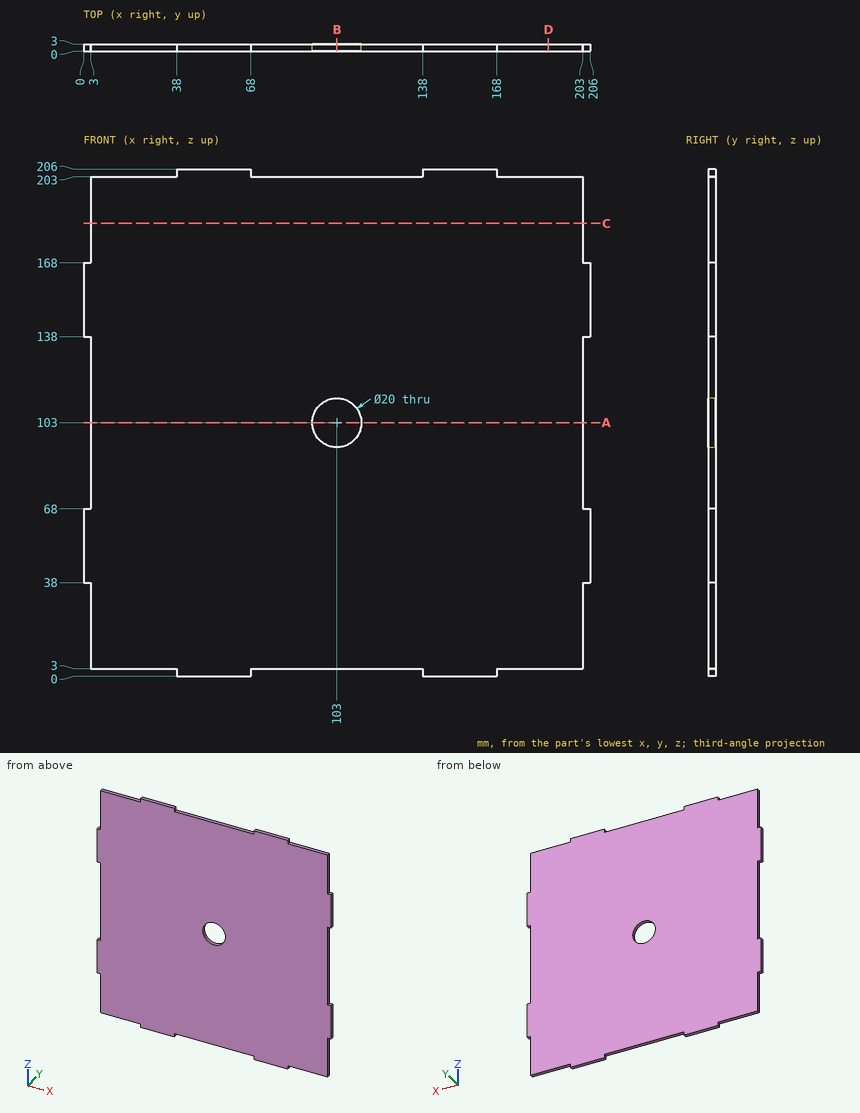
Job drawing, mm, ordinate dimensions from the low corner. One solid piece. Coordinates: 2 decimals unless noted, no trailing zeros. Order: outer loops, then holes, each group sorted by start corner. A loop starts at its lowest first (then second) coordinate and runs counter-clockwise, first axis right, second up. Notation, with made-up numbers: (60, 41.25) -> (109, 41.25) arc R32 ccw to (109, 76.25) -> close; hole circle Ø2 at (74, -21.5). An arc over 180 degrees is marked (long way). Answer in a Markdown table with one row per item. Add a question column.
Q1. Band-saw the part on C-C, the plane z = 184. List the corners of the cut face in (x, y).
Q2. Band-saw the part on D-D, the plane x = 189. List the corners of the cut face in (y, z).
Q3. Band-saw the part on B-B, the plane x = 103. List the corners of the cut face in (y, z), then the cut area to 3 significant figures.
Q4. Band-saw the part on A-A, the plane z = 103. List the corners of the cut face in (x, y).
Q5. Drop flat-ended pins along their axis: pin 1 (0.9 mm diameter, centred on y = 1.5, z = 1.5, fed in from +X); pin 2 (0.9 mm diameter, centred on y = 1, z = 1, fed in from -X); pin 3 (1.5 mm diameter, centred on x = 174, y = 1, fed in from +Z). Give the stop position or say it passes through.
Q6. Wall check: line 1 along X through (y, z) = (0.8, 103); line 2 along Z through (x, y) = (15.5, 1.25); line 3 along X through (y, z) = (1.7, 110). Give the ranges that are in metal, low to high. Write a range as [from, to].
Answers follow:
| question | item | result |
|---|---|---|
| 1 | outline | (3, 0) -> (203, 0) -> (203, 3) -> (3, 3) -> close |
| 2 | outline | (0, 3) -> (3, 3) -> (3, 203) -> (0, 203) -> close |
| 3 | outline | (0, 3) -> (3, 3) -> (3, 93) -> (0, 93) -> close; (0, 113) -> (3, 113) -> (3, 203) -> (0, 203) -> close |
| 3 | area | 540 mm^2 |
| 4 | outline | (3, 0) -> (93, 0) -> (93, 3) -> (3, 3) -> close; (113, 0) -> (203, 0) -> (203, 3) -> (113, 3) -> close |
| 5 | pin 1 | x = 168 |
| 5 | pin 2 | x = 38 |
| 5 | pin 3 | z = 203 |
| 6 | line 1 | [3, 93], [113, 203] |
| 6 | line 2 | [3, 203] |
| 6 | line 3 | [3, 95.86], [110.14, 203] |
